Geometry check sheet. Reference: the model listing, model coordinates, mm. Face numbers are marked on the shaded views. A direction names the side the tool comes from. Coordinates: 2 decimals unless noted, no trailing zeros. Write each loop counter-clockwise with the first axis right and the second up, starting at its lowest first coordinate (ties: lowest second). Pieces come first, ordered by that corner, then holes. Notation, with made-up numbers: (-38, -37) -> (2, -37) arc R7 cw to (2, -31) -> close; hole circle Ø2 at (41.5, 52.25). An arc over 180 degrees is marked (long way). One line per question, with ' | ' between items.
```python
from build123d import *

# Parameters (mm, degrees)
BOSS_EXTRUDE1_DEPTH             = 15.875
SKETCH2_W                       = 25.4
SKETCH2_H                       = 11.1125
CUT_EXTRUDE1_DEPTH              = 32.75
F_1_4_0_25_DIAMETER_HOLE1_D     = 6.35
F_1_4_0_25_DIAMETER_HOLE1_DEPTH = 44.45
F_1_4_0_25_DIAMETER_HOLE1_TIP   = 1.907732465
F_10_CLEARANCE_HOLE1_D          = 5.1054


with BuildPart() as part:
    # Sketch1 → Boss-Extrude1 (new body, symmetric)
    with BuildSketch(Plane.XY):
        Polygon((0, 0), (0, 25.4), (25.4, 25.4), (25.4, 0), (31.75, 0), (31.75, 31.75), (-31.75, 31.75), (-31.75, 0), align=None)
    extrude(amount=BOSS_EXTRUDE1_DEPTH, both=True)

    # Sketch2 → Cut-Extrude1 (cut, through all)
    with BuildSketch(Plane(origin=(0, 31.75, 0), x_dir=(1, 0, 0), z_dir=(0, 1, 0))):
        with Locations((-19.05, 0)):
            Rectangle(SKETCH2_W, SKETCH2_H)
    extrude(amount=-CUT_EXTRUDE1_DEPTH, mode=Mode.SUBTRACT)

    # 1/4 (0.25) Diameter Hole1
    with Locations(Plane(origin=(31.75, 0, 0), x_dir=(0, 0, -1), z_dir=(1, 0, 0))):
        with Locations((-9.525, 12.7), (9.525, 12.7)):
            Hole(F_1_4_0_25_DIAMETER_HOLE1_D / 2, depth=F_1_4_0_25_DIAMETER_HOLE1_DEPTH)
            with Locations((0, 0, -(F_1_4_0_25_DIAMETER_HOLE1_DEPTH + F_1_4_0_25_DIAMETER_HOLE1_TIP / 2))):  # 118° drill point
                Cone(0, F_1_4_0_25_DIAMETER_HOLE1_D / 2, F_1_4_0_25_DIAMETER_HOLE1_TIP, mode=Mode.SUBTRACT)

    # #10 Clearance Hole1 (through all)
    with Locations(Plane.XY.offset(15.875)):
        with Locations((-19.05, 12.7)):
            Hole(F_10_CLEARANCE_HOLE1_D / 2)


solid = part.part
```
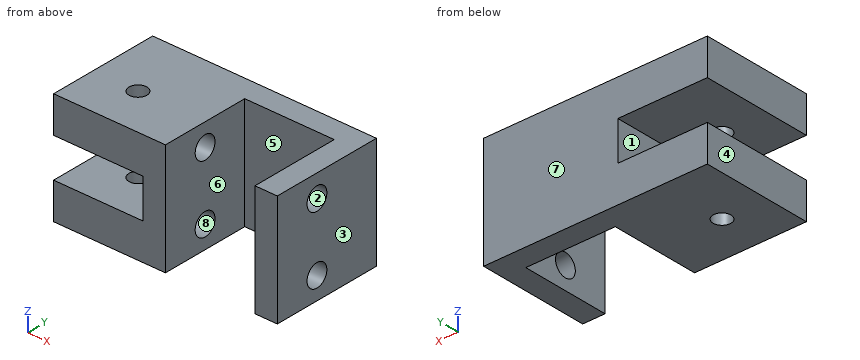
(1) Cross-section at C-C (z = -13.5). Record the cut outline in (x, y).
Answers below:
outline: (-31.75, 0) -> (0, 0) -> (0, 25.4) -> (25.4, 25.4) -> (25.4, 0) -> (31.75, 0) -> (31.75, 31.75) -> (-31.75, 31.75) -> close; hole circle Ø5.11 at (-19.05, 12.7)
(2) Depth check by flat-ended pin: P1, Ø4.5, axis at x = -19.05, y = 12.7, coming from the +Z side; P2, Ø5.5, axis at y = 14, z = -1, coming from the -X side; P3, Ø5.5, axis at y = 12.7, z = -9.525, coming from the +X side. Enter the tip coordinate at first touch or a pass-through.
Answers below:
P1: passes through | P2: stops at x = -6.35 | P3: stops at x = -12.96
(3) Cross-section at B-B (x = -19.05). Record the cut outline in (y, z) (3 decimals), plus the area to 3 significant figures.
Answers below:
outline: (0, -15.875) -> (10.147, -15.875) -> (10.147, -5.556) -> (0, -5.556) -> close; (0, 5.556) -> (10.147, 5.556) -> (10.147, 15.875) -> (0, 15.875) -> close; (15.253, -15.875) -> (31.75, -15.875) -> (31.75, -5.556) -> (15.253, -5.556) -> close; (15.253, 5.556) -> (31.75, 5.556) -> (31.75, 15.875) -> (15.253, 15.875) -> close | area: 550 mm²
(4) Cross-section at A-A (y = 20). Record the cut outline in (x, z) (3 decimals), plus the area to 3 significant figures.
Answers below:
outline: (-31.75, -15.875) -> (0, -15.875) -> (0, 15.875) -> (-31.75, 15.875) -> (-31.75, 5.556) -> (-6.35, 5.556) -> (-6.35, -5.556) -> (-31.75, -5.556) -> close; (25.4, -15.875) -> (31.75, -15.875) -> (31.75, 15.875) -> (25.4, 15.875) -> close | area: 927 mm²
(5) Tool access check on the marked faces 1, 2, 3, 4 and 5. Record the directions out of +Z, -Z, +X, -X, +Y, -Y that give a thin tool (end or side, any length) a straight path to the whole face; none if there is none.
Answers below:
face 1: -X, +Y, -Y | face 2: +X | face 3: +Z, -Z, +X, +Y, -Y | face 4: +Z, -Z, -X, +Y, -Y | face 5: +Z, -Z, -Y
(6) Material ranges on line 1 (X direction, y = 3.5, z = -12); line 2 (X direction, y = 21, z = -4); line 3 (Y direction, x = -19.05, z = -13.25), recorded low to high.
Answers below:
line 1: x = -31.75 to 0, 25.4 to 31.75 | line 2: x = -6.35 to 0, 25.4 to 31.75 | line 3: y = 0 to 10.15, 15.25 to 31.75
(7) Draft check along Y on the marked faces 6, 7 and 8. Enter one of: pulls with the +Y half, pulls with the -Y half, needs draft (parallel to the pull), parting line crosses it, or undercut.
Answers below:
face 6: needs draft | face 7: pulls with the +Y half | face 8: undercut
(8) Cross-section at D-D (x = -26.5). Record the cut outline in (y, z) (3 decimals).
Answers below:
outline: (0, -15.875) -> (31.75, -15.875) -> (31.75, -5.556) -> (0, -5.556) -> close; (0, 5.556) -> (31.75, 5.556) -> (31.75, 15.875) -> (0, 15.875) -> close
